from build123d import *

# Parameters (mm, degrees)
F1_DEPTH = 100
F2_ANGLE = 90
F4_ANGLE = 90
F5_DEPTH = 20.6729215554


with BuildPart() as f1:
    # F0 (on Front) → F1 (new body, symmetric)
    with BuildSketch(Plane.XZ):
        with BuildLine():
            ThreePointArc((50, 6.5869449865), (35.7017719302, 1.6669963579), (20.6729215554, 0))
            Line((20.6729215554, 0), (0, 0))
            Line((0, 0), (0, -4.4683294598))
            Line((0, -4.4683294598), (66.0657225847, -4.4683294598))
            Line((66.0657225847, -4.4683294598), (66.0657225847, 21.0250243545))
            Line((66.0657225847, 21.0250243545), (63.0657225847, 21.0250243545))
            ThreePointArc((63.0657225847, 21.0250243545), (57.9713766483, 12.5042019267), (50, 6.5869449865))
        make_face()
    extrude(amount=F1_DEPTH, both=True)

    # F1_face (on face) → F2 (revolve)
    with BuildSketch(Plane(origin=(44.1969490295, -100, 1.9928313496), x_dir=(1, 0, 0), z_dir=(0, -1, 0))):
        with BuildLine():
            Line((21.8687735552, -6.4611608094), (21.8687735552, 19.0321930048))
            Line((21.8687735552, 19.0321930048), (18.8687735552, 19.0321930048))
            ThreePointArc((18.8687735552, 19.0321930048), (13.7744276188, 10.511370577), (5.8030509705, 4.5941136369))
            ThreePointArc((5.8030509705, 4.5941136369), (-8.4951770993, -0.3258349918), (-23.5240274741, -1.9928313496))
            Line((-23.5240274741, -1.9928313496), (-44.1969490295, -1.9928313496))
            Line((-44.1969490295, -1.9928313496), (-44.1969490295, -6.4611608094))
            Line((-44.1969490295, -6.4611608094), (21.8687735552, -6.4611608094))
        make_face()
    revolve(axis=Axis((0, -100, -2.2341647299), (0, 0, -1)), revolution_arc=F2_ANGLE)

    # F3 (on face) → F4 (revolve)
    with BuildSketch(Plane(origin=(0, 100, 0), x_dir=(-1, 0, 0), z_dir=(0, 1, 0))):
        with BuildLine():
            Line((-63.0657225847, 21.0250243545), (-66.0657225847, 21.0250243545))
            Line((-66.0657225847, 21.0250243545), (-66.0657225847, -4.4683294598))
            Line((-66.0657225847, -4.4683294598), (-20.6729215554, -4.4683294598))
            Line((-20.6729215554, -4.4683294598), (-20.6729215554, 0))
            ThreePointArc((-20.6729215554, 0), (-35.7017719302, 1.6669963579), (-50, 6.5869449865))
            ThreePointArc((-50, 6.5869449865), (-57.9713766483, 12.5042019267), (-63.0657225847, 21.0250243545))
        make_face()
    revolve(axis=Axis((20.6729215554, 100, -2.2341647299), (0, 0, 1)), revolution_arc=F4_ANGLE)

    # F5 (add, through all): a face of the model
    f5_faces = [f1.faces().sort_by_distance(p)[0] for p in [
        (20.6729215554, 129.9863399133, 2.7995583272),
    ]]
    extrude(f5_faces, amount=F5_DEPTH)

    # F6: F1 across face


with BuildPart() as f1_1:
    add(f1.part)
    add(f1.part.mirror(Plane(origin=(0, -10.3364607777, 0.2594817433), x_dir=(0, -1, 0), z_dir=(-1, 0, 0))))


solid = f1_1.part
For this review, take the finished solid that the model builds, in its own axes (mm). A direction names the side the tool comes from. Round coordinates to 2 decimals unless told otherwise and drop trailing zeros. Order: outer loops, then holes, each group sorted by start corner. A loop starts at its lowest first (then second) coordinate and runs counter-clockwise, first axis right, second up. Notation, with made-up numbers: M 73,52 L 96,52 A23 cw 96,62 Z; hole C -34.75,27 d1. An arc over 180 degrees is marked long. Use a Markdown table: item, result. Add a question column.
Item 1: To check wall thickness, follow line 1 along Y through (x, z) = (0, -0.75); line 2 along Z through (x, y) = (6, -106.5); line 3 along X through (y, z) = (-132.5, 8.5). State the ranges of each line that lie inside material, in increasing order.
Item 2: Add section A-A, the plane y = -50. Give the boundary of the cut face in (x, z).
Item 3: Tool access review of faces 1 (the cylindrical face through (-1.45, -166.05, 8.46)), 2 (the cylindrical face through (35.909, -1.4, 1.714)): name each direction out of +Z, -Z, +X, -X, +Y, -Y from which nothing blocks a thin tool from reaching the whole face with its end or side.
Item 4: Insertion check: pin 1 (1.5 mm diameter, centred on x = 5.5, y = 7, fed in from +Z); pin 2 (2 mm diameter, centred on x = -40.5, z = 6, fed in from -Y); pin 3 (12 mm diameter, centred on x = 40.5, z = 13, fed in from +Y). Each pin has a flat end and moves straight along its axis. Give the tip position at first contact, or say it passes through.
Item 5: Mouldability with a two-part tool opening along Y and no side actions: class faces 3 (the cylindrical face through (-53.121, 131.743, 8.1)), 4 (the cylindrical face through (58.065, -1.4, 12.608)), 5 (the flat face through (66.066, -1, 8)) as released by +Y, released by -Y, zero draft, split by the parting line, or undercut.
Geometry results:
| question | item | result |
|---|---|---|
| 1 | line 1 | y = -166.07 to 145.39 |
| 1 | line 2 | z = -4.47 to 0 |
| 1 | line 3 | x = -57.52 to -42.32, 42.32 to 57.52 |
| 2 | outline | M -66.07,-4.47 L 66.07,-4.47 L 66.07,21.03 L 63.07,21.03 A25.4 cw 50,6.59 A68.58 cw 20.67,0 L -20.67,0 A68.58 cw -50,6.59 A25.4 cw -63.07,21.03 L -66.07,21.03 Z |
| 3 | face 1 | +Z, -Z, -Y |
| 3 | face 2 | +Z |
| 4 | pin 1 | stops at z = 0 |
| 4 | pin 2 | stops at y = -152.96 |
| 4 | pin 3 | stops at y = 143.24 |
| 5 | face 3 | released by +Y |
| 5 | face 4 | undercut |
| 5 | face 5 | zero draft |
